```python
from build123d import *

# Parameters (mm, degrees)
SKETCH1_W           = 19.05
SKETCH1_H           = 39.6875
BOSS_EXTRUDE1_DEPTH = 44.45
SHELL1_T            = -3.175
CUT_EXTRUDE1_REACH  = 51.601
SKETCH2_R           = 2.15265
FILLET2_R           = 6.35


with BuildPart() as part:
    # Sketch1 → Boss-Extrude1 (new body)
    with BuildSketch(Plane.XY):
        Rectangle(SKETCH1_W, SKETCH1_H)
    extrude(amount=-BOSS_EXTRUDE1_DEPTH)

    # Shell1
    shell1_openings = [part.faces().sort_by_distance(p)[0] for p in [
        (-9.525, 0, -22.225),
        (0, 19.84375, -22.225),
    ]]
    offset(amount=SHELL1_T, openings=shell1_openings, kind=Kind.INTERSECTION)

    # Sketch2 → Cut-Extrude1 (cut, up to next)
    with BuildSketch(Plane.XY, mode=Mode.PRIVATE) as cut_extrude1_sk1:
        with Locations((-3.175, -5.55625)):
            Circle(SKETCH2_R)
    cut_extrude1_tool1 = extrude(cut_extrude1_sk1.sketch, amount=-CUT_EXTRUDE1_REACH, mode=Mode.PRIVATE) & part.part
    # Sketch2 → Cut-Extrude1 (cut, up to next)
    with BuildSketch(Plane.XY, mode=Mode.PRIVATE) as cut_extrude1_sk2:
        with Locations((-3.175, 13.49375)):
            Circle(SKETCH2_R)
    cut_extrude1_tool2 = extrude(cut_extrude1_sk2.sketch, amount=-CUT_EXTRUDE1_REACH, mode=Mode.PRIVATE) & part.part
    add(cut_extrude1_tool1.solids().sort_by_distance((-3.175, -5.55625, 0))[0], mode=Mode.SUBTRACT)
    add(cut_extrude1_tool2.solids().sort_by_distance((-3.175, 13.49375, 0))[0], mode=Mode.SUBTRACT)

    # Fillet2
    fillet2_edges = [part.edges().sort_by_distance(p)[0] for p in [
        (-9.525, 19.84375, -1.5875),
    ]]
    fillet(fillet2_edges, radius=FILLET2_R)


solid = part.part
```
The model under review builds one solid part; all positions refer to its coordinate system, in mm. A direction names the side the tool comes from. Give positions to 0.01 mm unless a question says otherwise; leave off trailing zeros. Write each loop counter-clockwise with the first axis right and the second up, starting at its lowest first coordinate (ties: lowest second). Pieces come first, ordered by that corner, then holes. Notation, with made-up numbers: M 32.25,33 L 51.25,33 A14 cw 51.25,55 Z; hole C 49.25,-5 d9. An arc over 180 degrees is marked long. Write item = value, one per line. Start each with the question number.
Q1. We need section D-D (y = -6.5). State the section outline as (x, z) points (3 decimals), plus the area to 3 significant figures.
Q2. We need section B-B (y = 10). State the section outline as (x, z) points (3 decimals), plus the area to 3 significant figures.
Q3. Clearance check with flat-ended pins moving along their axes: pin 1 (6 mm diameter, centred on y = -0.5, z = -19.5, fed in from -X); pin 2 (2.5 mm diameter, centred on x = -3.18, y = -5.56, fed in from +Z) (3 decimals); pin 3 (2 mm diameter, centred on x = 2, z = -12, fed in from +Y). State where each tip first meets the part, or that it passes through.
Q4. Machinability: for faces 4 (the face through (-1.186, 12.669, -1.565)), 5 (the face through (-2, -16.669, -22)), 6 (the face through (-9.525, -18, -24)), 7 (the face through (-7.714, 17.934, -1.61)), which of the approach directions +Z, -Z, +X, -X, +Y, -Y give a long, thin tool a straight path to every point of the face, cutting with its end or side? Answer none if there is none.
Q5. We need section C-C (x = -4.5). State the section outline as (y, z) points (3 decimals), plus the area to 3 significant figures.
Q6. Mouldability with a two-part tool opening along X and no side actions: class faces 1 (the face through (6.35, 1, -22)), 2 (the face through (-2.182, -7.466, -1.565)), 3 (the face through (0, 0, -44.45)) as released by +X, released by -X, zero draft, split by the parting line, or undercut.
Q7. For line 1 (Z direction, x = -8.5, y = -8) (3 decimals); line 2 (X direction, y = 15.5, z = -18) (3 decimals); line 3 (Y direction, x = -5, z = -12), list the stretches that pass through material, from the lowest coordinate up.
Q8. We need section A-A (x = 5.25). State the section outline as (y, z) points (3 decimals).
Result set:
q1.outline = M -9.525,-44.45 L 9.525,-44.45 L 9.525,0 L -1.24,0 L -1.24,-3.175 L 6.35,-3.175 L 6.35,-41.275 L -9.525,-41.275 Z; M -9.525,-3.175 L -5.11,-3.175 L -5.11,0 L -9.525,0 Z
q1.area = 230 mm2
q2.outline = M -9.525,-44.45 L 9.525,-44.45 L 9.525,0 L -9.525,0 L -9.525,-3.175 L 6.35,-3.175 L 6.35,-41.275 L -9.525,-41.275 Z
q2.area = 242 mm2
q3.pin_1 = 6.35
q3.pin_2 = -41.275
q3.pin_3 = -16.67
q4.face_4 = +Z
q4.face_5 = -X, +Y
q4.face_6 = +Z, -Z, -X, +Y, -Y
q4.face_7 = +Z, -X, +Y
q5.outline = M -19.844,-44.45 L 19.844,-44.45 L 19.844,-41.275 L -16.669,-41.275 L -16.669,-3.175 L -7.253,-3.175 L -7.253,0 L -19.844,0 Z; M -3.86,-3.175 L 11.797,-3.175 L 11.797,0 L -3.86,0 Z; M 15.19,-3.175 L 19.704,-3.175 L 19.704,0 L 15.19,0 Z
q5.area = 351 mm2
q6.face_1 = released by -X
q6.face_2 = undercut
q6.face_3 = zero draft
q7.line_1 = -44.45 to -41.275, -3.175 to 0
q7.line_2 = 6.35 to 9.525
q7.line_3 = -19.84 to -16.67
q8.outline = M -19.844,-44.45 L 19.844,-44.45 L 19.844,-41.275 L -16.669,-41.275 L -16.669,-3.175 L 19.844,-3.175 L 19.844,0 L -19.844,0 Z
